Design review of the part built by this model. Coordinates are the model's own, in mm. Coordinates: 2 decimals unless noted, no trailing zeros. Loops run counter-clockwise (first coordinate to the right, second up) from the corner with the lowest first, then second, coordinate; pieces in that order, holes last. Notation, with made-up numbers: M 66.5,39 L 94.5,39 A17 ccw 94.5,68 Z; hole C -1.75,-10.5 d4. An arc over 180 degrees is marked long. Write item = value, one per line. Start each with the question number.
from build123d import *

# Parameters (mm, degrees)
F1_DEPTH = 0.127


# Not quite as in the source:
# - the program builds the solid bodies; features that only make, move or delete a surface that nothing else refers to are left out


with BuildPart() as f1:
    # F0 (on Top) → F1 (new body)
    with BuildSketch(Plane.XY):
        with BuildLine():
            Line((0, -2.6924), (0, 0))
            Line((0, 0), (0, 2.6924))
            ThreePointArc((0, 2.6924), (-0.3719743879, 3.5904256121), (-1.27, 3.9624))
            Line((-1.27, 3.9624), (-7.4879951317, 3.9624))
            ThreePointArc((-7.4879951317, 3.9624), (-7.9010514025, 4.0314484951), (-8.2691928483, 4.2310857998))
            Line((-8.2691928483, 4.2310857998), (-16.4196071517, 10.5898142002))
            ThreePointArc((-16.4196071517, 10.5898142002), (-16.7877485975, 10.7894515049), (-17.2008048683, 10.8585))
            Line((-17.2008048683, 10.8585), (-50.165, 10.8585))
            ThreePointArc((-50.165, 10.8585), (-51.0630256121, 10.4865256121), (-51.435, 9.5885))
            Line((-51.435, 9.5885), (-51.435, 0))
            Line((-51.435, 0), (-51.435, -9.5885))
            ThreePointArc((-51.435, -9.5885), (-51.0630256121, -10.4865256121), (-50.165, -10.8585))
            Line((-50.165, -10.8585), (-17.2008048683, -10.8585))
            ThreePointArc((-17.2008048683, -10.8585), (-16.7877485975, -10.7894515049), (-16.4196071517, -10.5898142002))
            Line((-16.4196071517, -10.5898142002), (-8.2691928483, -4.2310857998))
            ThreePointArc((-8.2691928483, -4.2310857998), (-7.9010514025, -4.0314484951), (-7.4879951317, -3.9624))
            Line((-7.4879951317, -3.9624), (-1.27, -3.9624))
            ThreePointArc((-1.27, -3.9624), (-0.3719743879, -3.5904256121), (0, -2.6924))
        make_face()
    extrude(amount=F1_DEPTH)


solid = f1.part
Q1. To check wall thickness, follow line 1 (Y direction, x = -4, z = 0.05); line 2 (X direction, y = 5.5, z = 0.05) (3 decimals); line 3 (X direction, y = 3.5, z = 0.05) (3 decimals). State the ranges of each line that lie inside material, in increasing order. Write a range as from..to.
Q2. Add section B-B on y = -6.75. State the section outline as (x, z) points (3 decimals).
Q3. Add section C-C on y = 7.75. State the section outline as (x, z) points (3 decimals).
Q4. Add section A-A on z = 0.05. State the section outline as (x, y) points (1 decimal).
Values follow:
q1.line_1 = -3.96..3.96
q1.line_2 = -51.435..-9.896
q1.line_3 = -51.435..-0.29
q2.outline = M -51.435,0 L -11.498,0 L -11.498,0.127 L -51.435,0.127 Z
q3.outline = M -51.435,0 L -12.78,0 L -12.78,0.127 L -51.435,0.127 Z
q4.outline = M -51.4,-9.6 A1.3 ccw -50.2,-10.9 L -17.2,-10.9 A1.3 ccw -16.4,-10.6 L -8.3,-4.2 A1.3 cw -7.5,-4 L -1.3,-4 A1.3 ccw 0,-2.7 L 0,2.7 A1.3 ccw -1.3,4 L -7.5,4 A1.3 cw -8.3,4.2 L -16.4,10.6 A1.3 ccw -17.2,10.9 L -50.2,10.9 A1.3 ccw -51.4,9.6 Z
